```python
from build123d import *

# Parameters (mm, degrees)
F3_R     = 1.5
F4_DEPTH = 12.5


with BuildPart() as f2:
    # F0 (on Front) → F2 (revolve)
    with BuildSketch(Plane.XZ):
        Polygon((7.5, 0), (1.5, 0), (1.5, -6), (3.175, -6), (3.175, -5), (4.175, -5), (4.175, -4), (7.5, -4), align=None)
    revolve(axis=Axis((0, 0, -5.151412), (0, 0, -1)))

    # F3 (on Front) → F4 (cut, symmetric)
    with BuildSketch(Plane.XZ):
        Circle(F3_R)
    extrude(amount=F4_DEPTH, both=True, mode=Mode.SUBTRACT)


solid = f2.part
```
For this review, take the finished solid that the model builds, in its own axes (mm). A direction names the side the tool comes from. Round coordinates to 2 decimals unless told otherwise and drop trailing zeros. Write each loop counter-clockwise with the first axis right and the second up, starting at its lowest first coordinate (ties: lowest second). Pieces come first, ordered by that corner, then holes. Notation, with made-up numbers: M 14.5,82.25 L 67.5,82.25 A25 cw 67.5,116.25 Z; hole C -21,-37 d10. An arc over 180 degrees is marked long. One line per item, written item: value. Start each with the question number.
(1) We need section A-A (x = 0). Give the boundary of the cut face in (y, z) (3 decimals), and give its area (3 significant figures).
(2) Insertion check: pin 1 (3.5 mm diameter, centred on x = 0, y = 0, fed in from -Z); pin 2 (2 mm diameter, centred on y = 2, z = -3, fed in from +X); pin 3 (1.5 mm diameter, centred on y = -3, z = -2.5, fed in from +X); pin 4 (2 mm diameter, centred on x = 1.5, z = -1.5, fed in from -Y). Each pin has a flat end and moves straight along its axis. Give the tip position at first contact, or say it passes through.
(3) We need section C-C (z = -5.25). Give the boundary of the cut face in (x, y) (3 decimals), and give its area (3 significant figures).
(4) Wall thickness on line 1 (X direction, y = 0, z = -3.3); line 2 (Z direction, x = 5, y = 3.5): over which ranges is each line inside the solid? List them lowest first.
(5) The part is to be moulded in two halves that separate along X. For faces 1 (the cylindrical face through (0, -4.6, -1.5)), 2 (the flat face through (-3.2, 3.2, -4)), 3 (the cylindrical face through (3.982, -1.254, -4.493)), say which applies: released by +X, released by -X, zero draft, split by the parting line, or undercut.
(6) We need section B-B (y = 0.25). Give the boundary of the cut face in (x, z), and give its area (3 significant figures).
(7) We need section D-D (x = -2). Give the boundary of the cut face in (y, z), and give its area (3 significant figures).
(8) Machinability: for faces 4 (the cylindrical face through (-0.69, 3.1, -5.49)), 5 (the cylindrical face through (-1.5, -0.07, -3.71)), which of the approach directions +Z, -Z, +X, -X, +Y, -Y give a long, thin tool a straight path to every point of the face, cutting with its end or side? Answer none if there is none.
Result:
1. outline: M -7.5,-4 L -4.175,-4 L -4.175,-5 L -3.175,-5 L -3.175,-6 L -1.5,-6 L -1.5,-1.5 L -7.5,-1.5 Z; M 1.5,-6 L 3.175,-6 L 3.175,-5 L 4.175,-5 L 4.175,-4 L 7.5,-4 L 7.5,-1.5 L 1.5,-1.5 Z
1. area: 38.7 mm²
2. pin 1: z = -6
2. pin 2: x = 7.43
2. pin 3: x = 7.15
2. pin 4: y = -7.48
3. outline: C 0,0 d6.35; hole C 0,0 d3
3. area: 24.6 mm²
4. line 1: -7.5 to -1.5, 1.5 to 7.5
4. line 2: -4 to 0
5. face 1: undercut
5. face 2: zero draft
5. face 3: split by the parting line
6. outline: M -7.5,-4 L -4.17,-4 L -4.17,-5 L -3.17,-5 L -3.17,-6 L -1.48,-6 L -1.48,-0.25 A1.5 cw -1.5,0 L -7.5,0 Z; M 1.48,-6 L 3.17,-6 L 3.17,-5 L 4.17,-5 L 4.17,-4 L 7.5,-4 L 7.5,0 L 1.5,0 A1.5 cw 1.48,-0.25 Z
6. area: 56.9 mm²
7. outline: M -7.23,-4 L -3.66,-4 L -3.66,-5 L -2.47,-5 L -2.47,-6 L 2.47,-6 L 2.47,-5 L 3.66,-5 L 3.66,-4 L 7.23,-4 L 7.23,0 L -7.23,0 Z
7. area: 70.1 mm²
8. face 4: -Z
8. face 5: +Z, -Z
